from build123d import *

# Parameters (mm, degrees)
SKETCH_1_R          = 1.5
SKETCH_1_R_2        = 12
EXTRUDE_1_DEPTH     = 5
SKETCH_2_W          = 5
SKETCH_2_H          = 20
EXTRUDE_2_DEPTH     = 34
FILLET_2_R          = 10
SKETCH_4_W          = 20
SKETCH_4_H          = 3
EXTRUDE_3_DEPTH     = 35.1
FILLET_3_R          = 1
SKETCH_5_W          = 20
SKETCH_5_H          = 3
EXTRUDE_4_DEPTH     = 30
RIB_1_REACH         = 83.986
SKETCH_8_WALL_W     = 182.719813126
SKETCH_8_WALL_H     = 5
SKETCH_9_R          = 2.5
CUT_EXTRUDE_1_DEPTH = 30
SKETCH_10_R         = 2.5
CUT_EXTRUDE_2_DEPTH = 30
SKETCH_11_R         = 2.5
CUT_EXTRUDE_3_DEPTH = 30
SKETCH_12_R         = 3
CUT_EXTRUDE_4_DEPTH = 1
SKETCH_13_R         = 4
CUT_EXTRUDE_5_DEPTH = 1
SKETCH_14_W         = 23.937452614
SKETCH_14_H         = 5.8
EXTRUDE_5_DEPTH     = 5
FILLET_4_R          = 3


with BuildPart() as part:
    # 草图1 → 凸台-拉伸1 (new body)
    # profile 1 of 2: a face of its own
    with BuildSketch(Plane.XY):
        Polygon((42.3, 0), (0, 0), (0, -42.3), (17.3, -63.8), (22.3, -63.8), (22.3, -43.8), (42.3, -43.8), (42.3, -42.3), align=None)
        with Locations((5.65, -36.65)):
            Circle(SKETCH_1_R, mode=Mode.SUBTRACT)
        with Locations((36.65, -36.65)):
            Circle(SKETCH_1_R, mode=Mode.SUBTRACT)
        with Locations((21.15, -21.15)):
            Circle(SKETCH_1_R_2, mode=Mode.SUBTRACT)
        with Locations((5.65, -5.65)):
            Circle(SKETCH_1_R, mode=Mode.SUBTRACT)
        with Locations((36.65, -5.65)):
            Circle(SKETCH_1_R, mode=Mode.SUBTRACT)
    # profile 2 of 2: a face of its own
    with BuildSketch(Plane.XY):
        Polygon((42.3, 0), (0, 0), (0, -42.3), (17.3, -63.8), (22.3, -63.8), (22.3, -43.8), (42.3, -43.8), (42.3, -42.3), align=None)
        with Locations((5.65, -36.65)):
            Circle(SKETCH_1_R, mode=Mode.SUBTRACT)
        with Locations((36.65, -36.65)):
            Circle(SKETCH_1_R, mode=Mode.SUBTRACT)
        with Locations((21.15, -21.15)):
            Circle(SKETCH_1_R_2, mode=Mode.SUBTRACT)
        with Locations((5.65, -5.65)):
            Circle(SKETCH_1_R, mode=Mode.SUBTRACT)
        with Locations((36.65, -5.65)):
            Circle(SKETCH_1_R, mode=Mode.SUBTRACT)
    extrude(amount=EXTRUDE_1_DEPTH)

    # 草图2 → 凸台-拉伸2 (add)
    with BuildSketch(Plane(origin=(0, 0, 0), x_dir=(-1, 0, 0), z_dir=(0, 0, -1))):
        with Locations((-19.8, -53.8)):
            Rectangle(SKETCH_2_W, SKETCH_2_H)
    extrude(amount=EXTRUDE_2_DEPTH)

    # 圆角2
    fillet_2_edges = [part.edges().sort_by_distance(p)[0] for p in [
        (17.3, -53.8, 0),
    ]]
    fillet(fillet_2_edges, radius=FILLET_2_R)

    # 草图4 → 凸台-拉伸3 (add)
    with BuildSketch(Plane.XY.offset(5)):
        with Locations((32.3, -42.3)):
            Rectangle(SKETCH_4_W, SKETCH_4_H)
    extrude(amount=EXTRUDE_3_DEPTH)

    # 圆角3
    fillet_3_edges = [part.edges().sort_by_distance(p)[0] for p in [
        (32.3, -40.8, 5),
    ]]
    fillet(fillet_3_edges, radius=FILLET_3_R)

    # 草图5 → 凸台-拉伸4 (add)
    with BuildSketch(Plane(origin=(0, -40.8, 0), x_dir=(1, 0, 0), z_dir=(0, 1, 0))):
        with Locations((32.3, -38.6)):
            Rectangle(SKETCH_5_W, SKETCH_5_H)
    extrude(amount=EXTRUDE_4_DEPTH)

    # 草图8 wall → 筋1 (add, up to next)
    with BuildSketch(Plane(origin=(32.3, -33.3, 33.375935793), x_dir=(0, -0.895662677282, -0.444734042461), z_dir=(0, 0.444734042461, -0.895662677282)), mode=Mode.PRIVATE) as rib_1_sk1:
        Rectangle(SKETCH_8_WALL_W, SKETCH_8_WALL_H)
    rib_1_tool1 = extrude(rib_1_sk1.sketch, amount=-RIB_1_REACH, mode=Mode.PRIVATE) - part.part
    add(rib_1_tool1.solids().sort_by_distance((32.3, -33.3, 33.375935793))[0])

    # 草图9 → 切除-拉伸1 (cut)
    with BuildSketch(Plane.XY.offset(40.1)):
        with Locations((32.3, -17.795537052)):
            Circle(SKETCH_9_R)
    extrude(amount=-CUT_EXTRUDE_1_DEPTH, mode=Mode.SUBTRACT)

    # 草图10 → 切除-拉伸2 (cut)
    with BuildSketch(Plane(origin=(0, -40.8, 0), x_dir=(1, 0, 0), z_dir=(0, 1, 0))):
        with Locations(Location((32.3, -17.555140143, 0), (0, 0, 270))):
            Circle(SKETCH_10_R)
    extrude(amount=-CUT_EXTRUDE_2_DEPTH, mode=Mode.SUBTRACT)

    # 草图11 → 切除-拉伸3 (cut)
    with BuildSketch(Plane.ZY.offset(-17.3)):
        with Locations((-22.658194914, -53.8)):
            Circle(SKETCH_11_R)
    extrude(amount=-CUT_EXTRUDE_3_DEPTH, mode=Mode.SUBTRACT)

    # 草图12 → 切除-拉伸4 (cut)
    with BuildSketch(Plane.XY.offset(5)):
        with Locations((5.65, -5.65)):
            Circle(SKETCH_12_R)
        with Locations((36.65, -5.65)):
            Circle(SKETCH_12_R)
        with Locations((5.65, -36.65)):
            Circle(SKETCH_12_R)
        with Locations((38.15, -39.419310808)):
            Circle(SKETCH_12_R)
    extrude(amount=-CUT_EXTRUDE_4_DEPTH, mode=Mode.SUBTRACT)

    # 草图13 → 切除-拉伸5 (cut)
    with BuildSketch(Plane.ZY.offset(-17.3)):
        with Locations((-22.658194914, -53.8)):
            Circle(SKETCH_13_R)
    extrude(amount=-CUT_EXTRUDE_5_DEPTH, mode=Mode.SUBTRACT)

    # 草图14 → 凸台-拉伸5 (add)
    with BuildSketch(Plane(origin=(22.3, 0, 0), x_dir=(0, 0, -1), z_dir=(1, 0, 0))):
        with Locations((6.968726307, -53.8)):
            Rectangle(SKETCH_14_W, SKETCH_14_H)
    extrude(amount=EXTRUDE_5_DEPTH)

    # 圆角4
    fillet_4_edges = [part.edges().sort_by_distance(p)[0] for p in [
        (26.05, -40.8, 37.1),
        (38.55, -40.8, 37.1),
        (34.8, -40.8, 33.375935793),
        (34.8, -33.300000001, 37.1),
        (29.8, -40.8, 33.375935793),
        (29.8, -33.300000001, 37.1),
        (22.3, -41.8, 5),
        (14.8, -43.8, 0),
    ]]
    fillet(fillet_4_edges, radius=FILLET_4_R)


solid = part.part
Can you work these out from the model? Positions are in its coordinate system, mm. A direction names the side the tool comes from. Coordinates: 2 decimals unless noted, no trailing zeros. Order: outer loops, then holes, each group sorted by start corner. A loop starts at its lowest first (then second) coordinate and runs counter-clockwise, first axis right, second up. Notation, with made-up numbers: M -39,72 L -18,72 A23 cw -18,81 Z; hole C -10,-37.75 d11. An arc over 180 degrees is marked long. Write item = value, one per line.
(1) Suppose I cut it at C-C on x = 36.65. Please give me the cut outline in (y, z).
Results are:
outline = M -43.8,0 L -38.15,0 L -38.15,4 L -42.02,4 L -42.02,5 L -39.8,5 A1 cw -40.8,6 L -40.8,29.65 L -40.57,29.77 L -40.57,34.1 A2.77 cw -37.8,36.87 L -26.26,36.87 L -25.8,37.1 L -10.8,37.1 L -10.8,40.1 L -43.8,40.1 Z; M -35.15,0 L -7.15,0 L -7.15,4 L -8.65,4 L -8.65,5 L -35.15,5 Z; M -4.15,0 L 0,0 L 0,5 L -2.65,5 L -2.65,4 L -4.15,4 Z
(2) I need wall thicknesses on line 1 along X through (y, z) = (-36.65, 3); line 2 along Y through (x, z) = (5.65, 2.3); line 3 along Y through (x, z) = (32, 38). Which ranges of each line are inside material? Lowest first, please. Write a range as [from, to].
Results are:
line_1 = [0, 4.15], [7.15, 35.15], [38.15, 42.3]
line_2 = [-49.32, -38.15], [-35.15, -7.15], [-4.15, 0]
line_3 = [-43.8, -20.28], [-15.31, -10.8]
(3) Suppose I cut it at A-A on y = -21.15. Please give me the cut outline in (x, z).
Results are:
outline = M 0,0 L 9.15,0 L 9.15,5 L 0,5 Z; M 22.3,37.1 L 42.3,37.1 L 42.3,40.1 L 22.3,40.1 Z; M 33.15,0 L 42.3,0 L 42.3,5 L 33.15,5 Z
(4) Suppose I cut it at D-D on z = -23. Please give me the cut outline in (x, y).
Results are:
outline = M 17.3,-63.8 L 22.3,-63.8 L 22.3,-56.28 L 18.3,-56.28 L 18.3,-57.79 L 17.3,-57.79 Z; M 17.3,-49.81 L 18.3,-49.81 L 18.3,-51.32 L 22.3,-51.32 L 22.3,-43.8 L 17.3,-43.8 Z
(5) For pin 1 Ø8 at (x, y) = (5.65, -36.65) entering from +Z; pin 2 Ø3.5 at (x, z) = (33.5, 38.5) entering from +Y; pin 3 Ø1.5 at (y, z) = (-34.5, 33) entering from +X, each with a flat end and sliding along its axis, tell me the tip position at first contact or that it passes through.
Results are:
pin_1 = 5
pin_2 = -10.8
pin_3 = 34.8
(6) If we mould it in two halves opening along Z, with no side actions, what happens to faces 1 (the face through (16.57, -42.49, -0.52)), 2 (the face through (32.223, -33.195, 33.428)), 3 (the face through (38, -5, 2))? For each: pulls with the +Z half, pulls with the -Z half, needs draft (parallel to the pull), parting line crosses it, or undercut.
Results are:
face_1 = pulls with the -Z half
face_2 = undercut
face_3 = needs draft
(7) For faces 4 (the face through (32, -21, 37.1)), 5 (the face through (5, -39.58, 4.51)), 6 (the face through (38, -40, 4)), which set-ups out of +Z, -Z, +X, -X, +Y, -Y let a thin tool reach every point of the face, with its end or its side?
Results are:
face_4 = +Y
face_5 = +Z
face_6 = none
(8) Suppose I cut it at B-B on x = 13. Please give me the cut outline in (y, z), plus the area to 3 significant figures.
Results are:
outline = M -58.46,-1.78 L -43.54,-1.78 A3 cw -40.8,0 L -29.96,0 L -29.96,5 L -58.46,5 Z; M -12.34,0 L 0,0 L 0,5 L -12.34,5 Z
area = 232 mm2
